The listing builds one solid part. Answer for the finished solid, in the listing's coordinates (mm). Face numbers are marked on the shaded views. A direction names the side the tool comes from. Coordinates: 2 decimals unless noted, no trailing zeros. Write each loop counter-clockwise with the first axis right and the second up, starting at its lowest first coordinate (ties: lowest second). Pieces come first, ordered by that corner, then holes.
from build123d import *

# Parameters (mm, degrees)
F2_R     = 0.25
F3_SIZE  = 0.5
F4_SIZE  = 1
F6_DEPTH = 5


with BuildPart() as f1:
    # F0 (on Top) → F1 (revolve)
    with BuildSketch(Plane.XY):
        Polygon((0, 31), (0, 0), (6.5, 0), (6.5, 7.5), (4, 7.5), (4, 26), (2.975, 26), (2.975, 31), align=None)
    revolve(axis=Axis((0, 15.5, 0), (0, -1, 0)))

    # F2
    f2_edges = [f1.edges().sort_by_distance(p)[0] for p in [
        (-4, 7.5, 0),
        (-2.975, 26, 0),
    ]]
    fillet(f2_edges, radius=F2_R)

    # F3
    f3_edges = [f1.edges().sort_by_distance(p)[0] for p in [
        (-2.975, 31, 0),
    ]]
    chamfer(f3_edges, length=F3_SIZE)

    # F4
    f4_edges = [f1.edges().sort_by_distance(p)[0] for p in [
        (-6.5, 0, 0),
    ]]
    chamfer(f4_edges, length=F4_SIZE)

    # F5 (on face) → F6 (cut)
    with BuildSketch(Plane.XZ):
        Polygon((-3, 1.732051), (-3, -1.732051), (0, -3.464102), (3, -1.732051), (3, 1.732051), (0, 3.464102), align=None)
    extrude(amount=-F6_DEPTH, mode=Mode.SUBTRACT)


solid = f1.part
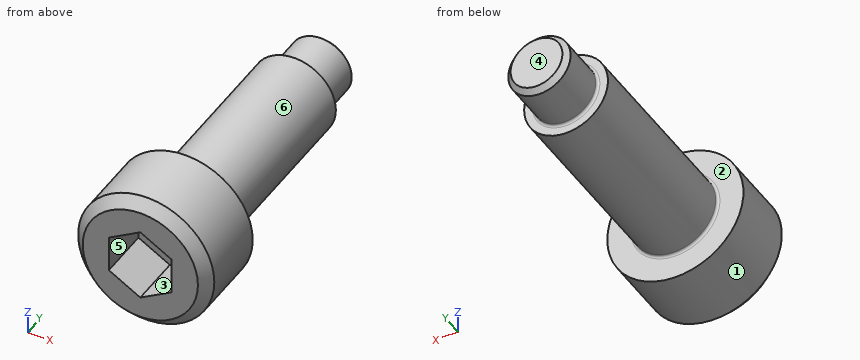
1. Section A-A on z = 0 is taken. Give the vertices of the cut face in (x, y) (3 decimals), then the cut area to 3 significant figures.
Results found:
outline: (-6.5, 1) - (-5.5, 0) - (-3, 0) - (-3, 5) - (3, 5) - (3, 0) - (5.5, 0) - (6.5, 1) - (6.5, 7.5) - (4.25, 7.5) arc R0.25 cw to (4, 7.75) - (4, 26) - (3.225, 26) arc R0.25 cw to (2.975, 26.25) - (2.975, 30.5) - (2.475, 31) - (-2.475, 31) - (-2.975, 30.5) - (-2.975, 26.25) arc R0.25 cw to (-3.225, 26) - (-4, 26) - (-4, 7.75) arc R0.25 cw to (-4.25, 7.5) - (-6.5, 7.5) - close
area: 244 mm2
2. Section B-B on y = 7 is taken. Give the vertices of the cut face in (x, z), then the cut area to 3 significant figures.
Results found:
outline: circle Ø13 at (0, 0)
area: 133 mm2
3. Flat-ended cylindrical pins translate along their axes: P1, Ø2, axis at x = -5, z = 5, coming from the +Y side; P2, Ø1.5, axis at x = -3.5, z = 3, coming from the +Y side; P3, Ø1.5, axis at y = 9.5, z = -0.5, coming from the +X side. Find the tip coordinate at first contact, or state that the pin passes through.
Results found:
P1: stops at y = 7.5
P2: stops at y = 26
P3: stops at x = 4
4. A tool of negligible diameter and unlimited length cuts with its end or side. For the marked faces 1, 2 and 3, from which of +Z, -Z, +X, -X, +Y, -Y can it reach the whole face along a straight path? Write none if from no direction.
Results found:
face 1: +Y, -Y
face 2: +Y
face 3: -Y
5. For a pull along X with two mould halves and no side action, classify the marked faces 4, 5 and 6 as pulls with the +X half, pulls with the -X half, needs draft (parallel to the pull), parting line crosses it, or undercut.
Results found:
face 4: needs draft
face 5: undercut
face 6: parting line crosses it
6. Section C-C on y = 10.5 is taken. Give the vertices of the cut face in (x, z), then the cut area to 3 significant figures.
Results found:
outline: circle Ø8 at (0, 0)
area: 50.3 mm2
7. Find the intervals of material crossed by L1, parallel to Y at x = 2.25, z = -3.75; L2, parallel to Y at x = 0.5, z = 0; L3, parallel to X at y = 3.5, z = 1.5, in increasing order.
Results found:
L1: y = 0 to 7.5
L2: y = 5 to 31
L3: x = -6.32 to -3, 3 to 6.32
